CAD build for the part. Positions are in the model's coordinates, mm. Face numbers are marked on the shaded views. A direction names the side the tool comes from. Coordinates: 2 decimals unless noted, no trailing zeros. Loops run counter-clockwise (first coordinate to the right, second up) from the corner with the lowest first, then second, coordinate; pieces in that order, holes last. Notation, with made-up numbers: (-3.75, 81.25) -> (51.25, 81.25) arc R19 ccw to (51.25, 100.25) -> close; hole circle Ø6 at (61, 19.25). An arc over 180 degrees is marked (long way). Answer as a JSON object with one key per item and string values. Group by question number.
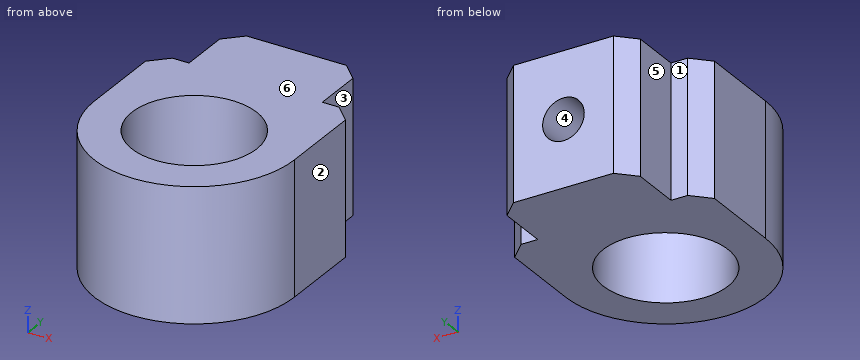
from build123d import *

# Parameters (mm, degrees)
SKETCH1_R           = 3.75
BOSS_EXTRUDE2_DEPTH = 8
SKETCH11_R          = 1.25
CUT_EXTRUDE5_DEPTH  = 5
CHAMFER1_SIZE       = 1


with BuildPart() as part:
    # Sketch1 → Boss-Extrude2 (new body)
    with BuildSketch(Plane.XY):
        with BuildLine():
            Line((-6, 0), (-6, 6))
            Line((-6, 6), (-4, 6))
            Line((-4, 6), (-4, 10))
            Line((-4, 10), (4, 10))
            Line((4, 10), (4, 6))
            Line((4, 6), (6, 6))
            Line((6, 6), (6, 0))
            ThreePointArc((6, 0), (0, -6), (-6, 0))
        make_face()
        Circle(SKETCH1_R, mode=Mode.SUBTRACT)
    extrude(amount=BOSS_EXTRUDE2_DEPTH)

    # Sketch11 → Cut-Extrude5 (cut)
    with BuildSketch(Plane(origin=(0, 10, 0), x_dir=(1, 0, 0), z_dir=(0, 1, 0))):
        with Locations(Location((0, -4, 0), (0, 0, 270))):
            Circle(SKETCH11_R)
    extrude(amount=-CUT_EXTRUDE5_DEPTH, mode=Mode.SUBTRACT)

    # Chamfer1
    chamfer1_edges = [part.edges().sort_by_distance(p)[0] for p in [
        (-6, 6, 4),
        (-4, 10, 4),
        (4, 10, 4),
        (6, 6, 4),
    ]]
    chamfer(chamfer1_edges, length=CHAMFER1_SIZE)


solid = part.part
Item 1: Band-saw the part on D-D, the plane y = 7.5. List the corners of the cut face in (x, z).
Item 2: Drill centre lines: L1, parallel to X at y = 8.55, z = 4; L2, parallel to Z at x = 0.75, y = 6.25; L3, parallel to Y at x = 0, z = 5. Where is each one in solid material? Low to high.
Item 3: Band-saw the part on C-C, the plane z = 6.75. List the corners of the cut face in (x, y), and give its area (3 significant figures).
Item 4: Flat gauge pins, fed straight in: P1, Ø1, axis at y = -3.5, z = 6, coming from the +X side; P2, Ø1, axis at y = -1, z = 3.5, coming from the +X side; P3, Ø3, axis at x = 4, z = 4, coming from the -Y side; P4, Ø7, axis at x = 0, y = 0, coming from the +Z side. Where does each tip first touch, or does it go through?
Item 5: Pull direction X, two halves, no side cores. Call the marked faces 4, 5 and 6: +X half, -X half, draft (parallel to the pull), parting line (faces both ways), or undercut.
Item 6: Band-saw the part on B-B, the plane y = 3. List the corners of the cut face in (x, z).
Item 7: 3-axis set-ups, long thin cutter, end or side, ignore diameter. For the marked faces 1, 2 and 3: which of +Z, -Z, +X, -X, +Y, -Y reach the whole face in a straight line?
Item 8: Band-saw the part on A-A, the plane x = 0. List the corners of the cut face in (y, z), and give its area (3 significant figures).
Reply:
{
 "1": {"outline": "(-4, 0) -> (4, 0) -> (4, 8) -> (-4, 8) -> close; hole circle Ø2.5 at (0, 4)"},
 "2": {"L1": "-4 to -1.25, 1.25 to 4", "L2": "0 to 3, 5 to 8", "L3": "-6 to -3.75, 3.75 to 5"},
 "3": {"outline": "(-6, 0) arc R6 ccw to (6, 0) -> (6, 5) -> (5, 6) -> (4, 6) -> (4, 9) -> (3, 10) -> (-3, 10) -> (-4, 9) -> (-4, 6) -> (-5, 6) -> (-6, 5) -> close; hole circle Ø7.5 at (0, 0)", "area": "114 mm²"},
 "4": {"P1": "x = 5.2", "P2": "x = 5.98", "P3": "y = -5.45", "P4": "through"},
 "5": {"face 4": "undercut", "face 5": "-X half", "face 6": "draft"},
 "6": {"outline": "(-6, 0) -> (-2.25, 0) -> (-2.25, 8) -> (-6, 8) -> close; (2.25, 0) -> (6, 0) -> (6, 8) -> (2.25, 8) -> close"},
 "7": {"face 1": "+Z, -Z, -X, +Y", "face 2": "+Z, -Z, +X, +Y, -Y", "face 3": "+Z, -Z, +X, +Y"},
 "8": {"outline": "(-6, 0) -> (-3.75, 0) -> (-3.75, 8) -> (-6, 8) -> close; (3.75, 0) -> (10, 0) -> (10, 2.75) -> (5, 2.75) -> (5, 5.25) -> (10, 5.25) -> (10, 8) -> (3.75, 8) -> close", "area": "55.5 mm²"}
}
